Could you check a few things on this model? Use its own coordinates, in mm. Round coordinates to 2 decimals unless told otherwise and drop trailing zeros. Write each loop counter-clockwise with the first axis right and the second up, starting at its lowest first coordinate (ties: lowest second). Pieces come first, ordered by that corner, then holes. Notation, with made-up numbers: (-13.75, 59) -> (20.25, 59) arc R22 ccw to (20.25, 86) -> close; hole circle Ø6 at (15.5, 46.5). An arc over 180 degrees is marked (long way). Answer as CSV lines item,"result". Start each with the question number.
Q1. If we mould it in two halves opening along X, with no side actions, what happens to faces 1 (the flat face through (-1, 1, 0)), 2 (the cylindrical face through (17.014, -61.4, 1.568))? For each: pulls with the +X half, pulls with the -X half, needs draft (parallel to the pull), parting line crosses it, or undercut.
Q2. Imagine slicing it at D-D on z = 1.6. Give the number of separate pieces and of enclosed holes in the cut face, and give its area (3 significant figures).
Q3. Imagine slicing it at C-C on y = 24. Please give me the cut outline in (x, z), and give its area (3 significant figures).
Q4. Imagine slicing it at B-B on x = -22. Please give me the cut outline in (y, z), and give its area (3 significant figures).
Q5. Will these pins go through, and if not, where does the flat tip stop? pin 1 Ø1.6 at (x, z) = (88.5, 1) entering from +Y (3 decimals); pin 2 Ø1.5 at (y, z) = (70, 2.5) entering from -X; pin 3 Ø1.6 at (y, z) = (87.5, 2) entering from +X.
Q6. Imagine slicing it at A-A on x = 69.5. Please give me the cut outline in (y, z), and give its area (3 significant figures).
Q7. If I drill on line 1 (Y direction, x = 38, z = 1.5); line 2 (Y direction, x = 5, z = 1.5); line 3 (X direction, y = -33, z = 1.2), over which ranges is the centre line in solid material (lowest first)? Write a range as [from, to].
from build123d import *

# Parameters (mm, degrees)
SKETCH3_W           = 180
SKETCH3_H           = 180
SKETCH3_R           = 3.875
SKETCH3_W_2         = 20
SKETCH3_H_2         = 3.18
SKETCH3_W_3         = 19.75
SKETCH3_W_4         = 60
SKETCH3_H_3         = 15
BOSS_EXTRUDE1_DEPTH = 3.18
CUT_EXTRUDE1_DEPTH  = 128.318939675
SKETCH5_R           = 1.436023081
SKETCH5_W           = 3.18
SKETCH5_H           = 80.125
CUT_EXTRUDE2_DEPTH  = 128.318939675


with BuildPart() as part:
    # Sketch3 → Boss-Extrude1 (new body)
    with BuildSketch(Plane.XY):
        Rectangle(SKETCH3_W, SKETCH3_H)
        with Locations(Location((13.938719016, -63.758151241, 0), (0, 0, 180))):
            Circle(SKETCH3_R, mode=Mode.SUBTRACT)
        with Locations((-28.286899392, 36.024803222)):
            Rectangle(SKETCH3_W_2, SKETCH3_H_2, mode=Mode.SUBTRACT)
        with Locations((-0.125, -46.269729843)):
            Rectangle(SKETCH3_W_3, SKETCH3_H_2, mode=Mode.SUBTRACT)
        with Locations((56.112903479, -67.514680034)):
            Rectangle(SKETCH3_W_4, SKETCH3_H_3, mode=Mode.SUBTRACT)
    extrude(amount=BOSS_EXTRUDE1_DEPTH)

    # Sketch4 → Cut-Extrude1 (cut, through all)
    with BuildSketch(Plane.XY.offset(3.18)):
        Polygon((1.5, 86.82), (10, 86.82), (10, 90), (-10, 90), (-10, 86.82), (-1.5, 86.82), (-1.5, 82.82), (-3.5, 82.82), (-3.5, 79.82), (-1.5, 79.82), (-1.5, 77), (1.5, 77), (1.5, 79.82), (3.5, 79.82), (3.5, 82.82), (1.5, 82.82), align=None)
        Polygon((1.5, -79.82), (1.5, -77), (-1.5, -77), (-1.5, -79.82), (-3.5, -79.82), (-3.5, -82.82), (-1.5, -82.82), (-1.5, -86.82), (-10, -86.82), (-10, -90), (10, -90), (10, -86.82), (1.5, -86.82), (1.5, -82.82), (3.5, -82.82), (3.5, -79.82), align=None)
    extrude(amount=-CUT_EXTRUDE1_DEPTH, mode=Mode.SUBTRACT)

    # Sketch5 → Cut-Extrude2 (cut, through all)
    with BuildSketch(Plane.XY.offset(3.18)):
        with Locations((-88, 0)):
            Circle(SKETCH5_R)
        with Locations((88, 0)):
            Circle(SKETCH5_R)
        with Locations((-88.41, 49.9375)):
            Rectangle(SKETCH5_W, SKETCH5_H)
        with Locations((-88.41, -49.9375)):
            Rectangle(SKETCH5_W, SKETCH5_H)
        with Locations((88.41, -49.9375)):
            Rectangle(SKETCH5_W, SKETCH5_H)
        with Locations((88.41, 49.9375)):
            Rectangle(SKETCH5_W, SKETCH5_H)
    extrude(amount=-CUT_EXTRUDE2_DEPTH, mode=Mode.SUBTRACT)


solid = part.part
Checks:
1,face 1,"needs draft"
1,face 2,"undercut"
2,separate pieces,"1"
2,enclosed holes,"6"
2,area,"30,100 mm^2"
3,outline,"(-86.82, 0) -> (86.82, 0) -> (86.82, 3.18) -> (-86.82, 3.18) -> close"
3,area,"552 mm^2"
4,outline,"(-90, 0) -> (34.43, 0) -> (34.43, 3.18) -> (-90, 3.18) -> close; (37.61, 0) -> (90, 0) -> (90, 3.18) -> (37.61, 3.18) -> close"
4,area,"562 mm^2"
5,pin 1,"y = 9.875"
5,pin 2,"x = -86.82"
5,pin 3,"x = 86.82"
6,outline,"(-90, 0) -> (-75.01, 0) -> (-75.01, 3.18) -> (-90, 3.18) -> close; (-60.01, 0) -> (90, 0) -> (90, 3.18) -> (-60.01, 3.18) -> close"
6,area,"525 mm^2"
7,line 1,"[-90, -75.01], [-60.01, 90]"
7,line 2,"[-86.82, -47.86], [-44.68, 86.82]"
7,line 3,"[-86.82, 86.82]"
